```python
from build123d import *

# Parameters (mm, degrees)
CROQUIS1_W              = 65
CROQUIS1_H              = 65
CROQUIS1_R              = 22.5
CROQUIS1_R_2            = 1.5
CROQUIS1_R_3            = 1.25
SALIENTE_EXTRUIR1_DEPTH = 2
REDONDEO1_R             = 15


with BuildPart() as part:
    # Croquis1 → Saliente-Extruir1 (new body)
    with BuildSketch(Plane.XY):
        Rectangle(CROQUIS1_W, CROQUIS1_H)
        Circle(CROQUIS1_R, mode=Mode.SUBTRACT)
        with Locations((0, 26)):
            Circle(CROQUIS1_R_2, mode=Mode.SUBTRACT)
        with Locations((26, 0)):
            Circle(CROQUIS1_R_2, mode=Mode.SUBTRACT)
        with Locations((0, -26)):
            Circle(CROQUIS1_R_2, mode=Mode.SUBTRACT)
        with Locations((-26, 0)):
            Circle(CROQUIS1_R_2, mode=Mode.SUBTRACT)
        with Locations((12.02081528, 28.991378029)):
            Circle(CROQUIS1_R_3, mode=Mode.SUBTRACT)
        with Locations(Location((28.991378029, 12.02081528, 0), (0, 0, 180))):
            Circle(CROQUIS1_R_3, mode=Mode.SUBTRACT)
        with Locations(Location((12.02081528, -28.991378029, 0), (0, 0, 180))):
            Circle(CROQUIS1_R_3, mode=Mode.SUBTRACT)
        with Locations((28.991378029, -12.02081528)):
            Circle(CROQUIS1_R_3, mode=Mode.SUBTRACT)
        with Locations(Location((-28.991378029, -12.02081528, 0), (0, 0, 180))):
            Circle(CROQUIS1_R_3, mode=Mode.SUBTRACT)
        with Locations((-12.02081528, -28.991378029)):
            Circle(CROQUIS1_R_3, mode=Mode.SUBTRACT)
        with Locations(Location((-12.02081528, 28.991378029, 0), (0, 0, 180))):
            Circle(CROQUIS1_R_3, mode=Mode.SUBTRACT)
        with Locations((-28.991378029, 12.02081528)):
            Circle(CROQUIS1_R_3, mode=Mode.SUBTRACT)
    extrude(amount=SALIENTE_EXTRUIR1_DEPTH)

    # Redondeo1
    redondeo1_edges = [part.edges().sort_by_distance(p)[0] for p in [
        (-32.5, 32.5, 1),
        (32.5, 32.5, 1),
        (32.5, -32.5, 1),
        (-32.5, -32.5, 1),
    ]]
    fillet(redondeo1_edges, radius=REDONDEO1_R)


solid = part.part
```
Work out the finished part from the listing and answer in its coordinate system (mm). Round coordinates to 2 decimals unless told otherwise and drop trailing zeros. Write each loop counter-clockwise with the first axis right and the second up, starting at its lowest first coordinate (ties: lowest second). Pieces come first, ordered by that corner, then holes.
1) A cutting plane is placed at D-D on x = 26. Determine the outline of the cut face in (y, z), and give its area (3 significant figures).
2) Consider probe 1 along X at (y, z) = (11, 0.2); probe 2 along Y at (x, z) = (8, 0.9); probe 3 along Y at (x, z) = (-17.5, 0.75). Determine where each line is inside the solid, lowest interval first.
3) Flat-ended cylindrical pins translate along their axes: P1, Ø1, axis at x = -21, z = 1, coming from the +Y side; P2, Ø4, axis at x = 0, y = 26, coming from the +Z side. Find the tip coordinate at first contact, or state that the pin passes through.
4) A cutting plane is placed at C-C on z = 1.1. Give the number of separate pieces and of enclosed holes in the cut face, and give its area (3 significant figures).
5) A cutting plane is placed at A-A on x = 0. Determine the outline of the cut face in (y, z).
6) Determine the mould class of faces 1 (the face through (27.99, -28.22, 1.01)), 2 (the face through (-27.5, 0.07, 0.99)), 3 (the face through (-22, 8, 0)) for opening direction X: pulls with the +X half, pulls with the -X half, needs draft (parallel to the pull), parting line crosses it, or undercut.
Entries:
1. outline: (-29.86, 0) - (-1.5, 0) - (-1.5, 2) - (-29.86, 2) - close; (1.5, 0) - (29.86, 0) - (29.86, 2) - (1.5, 2) - close
1. area: 113 mm2
2. probe 1: x = -32.5 to -29.71, -28.27 to -19.63, 19.63 to 28.27, 29.71 to 32.5
2. probe 2: y = -32.5 to -21.03, 21.03 to 32.5
2. probe 3: y = -32.5 to -14.14, 14.14 to 32.5
3. P1: stops at y = 32.2
3. P2: stops at z = 2
4. separate pieces: 1
4. enclosed holes: 13
4. area: 2,370 mm2
5. outline: (-32.5, 0) - (-27.5, 0) - (-27.5, 2) - (-32.5, 2) - close; (-24.5, 0) - (-22.5, 0) - (-22.5, 2) - (-24.5, 2) - close; (22.5, 0) - (24.5, 0) - (24.5, 2) - (22.5, 2) - close; (27.5, 0) - (32.5, 0) - (32.5, 2) - (27.5, 2) - close
6. face 1: pulls with the +X half
6. face 2: undercut
6. face 3: needs draft
